Answer from the drawing. Dimensions are ordinates in mm from the lowest x, y and z of the part. Give positions to 0.01 mm unless a question says otherwise; leave off trailing zeros. Order: outer loops, then holes, each group sorted by start corner. A loop starts at its lowest first (then second) coordinate and runs counter-clockwise, first axis right, second up. Notation, with made-up numbers: (2, 38.25) -> (21, 38.25) arc R14 ccw to (21, 52.25) -> close; hole circle Ø11 at (25, 81). An arc over 180 degrees is marked (long way). Write item = value, one per line. Start each with the question number.
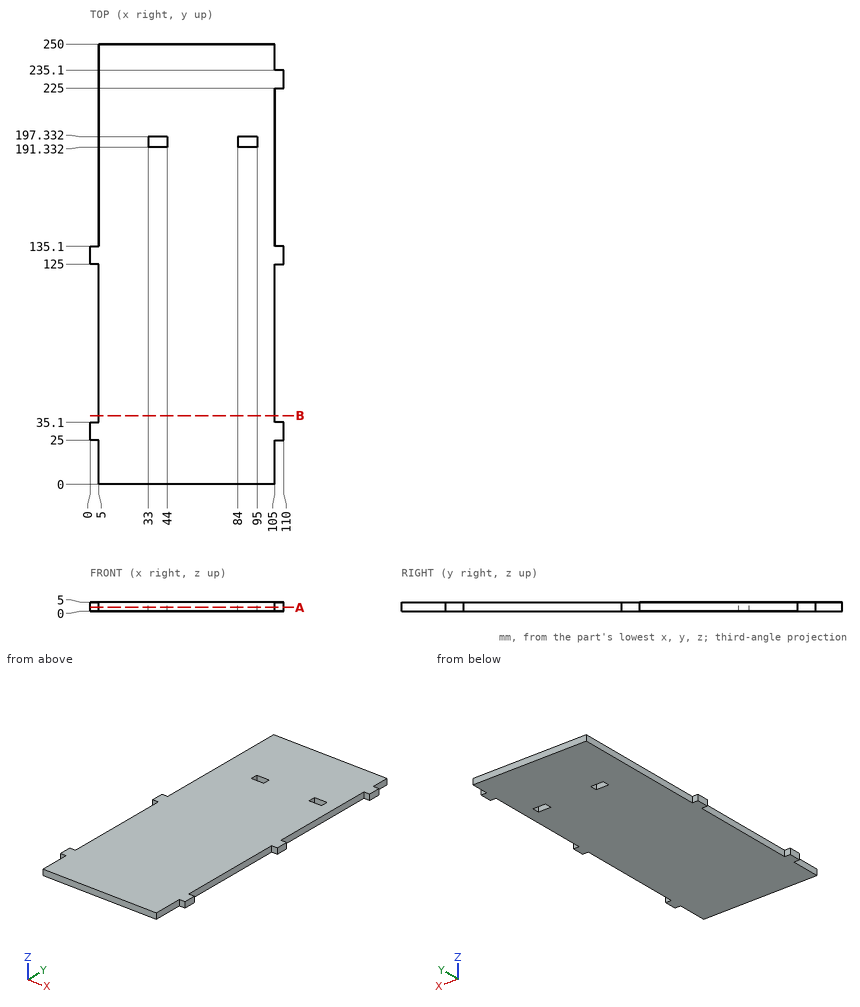
Item 1: Flat-ended cylindrical pins translate along their axes: pin 1 (1.5 mm diameter, centred on y = 196, z = 3, fed in from +X); pin 2 (1.5 mm diameter, centred on x = 2.5, z = 3, fed in from -Y); pin 3 (1.5 mm diameter, centred on y = 194.5, z = 2.5, fed in from -X); pin 4 (1 mm diameter, centred on x = 73.5, y = 164.5, fed in from -Z). Find the tip coordinate at first contact, or state that the pin passes through.
Item 2: A cutting plane is placed at B-B, the plane y = 39. Write down the section's boundary in (x, z).
Item 3: Consider L1, parallel to Y at x = 43, z = 3.35; L2, parallel to Y at x = 105.5, z = 0.7; L3, parallel to X at y = 177.5, z = 4.1. Determine where each line is inside the solid, lowest interval first. Write a range as from..to.
Item 4: A cutting plane is placed at A-A, the plane z = 2.15. Count the separate pieces of the cut face and the enclosed holes in it, plus the area to 3 significant figures.
Check values:
q1.pin_1 = 105
q1.pin_2 = 25
q1.pin_3 = 5
q1.pin_4 = 0
q2.outline = (5, 0) -> (105, 0) -> (105, 5) -> (5, 5) -> close
q3.L1 = 0..191.33, 197.33..250
q3.L2 = 25..35.1, 125..135.1, 225..235.1
q3.L3 = 5..105
q4.separate_pieces = 1
q4.enclosed_holes = 2
q4.area = 25,100 mm^2
